For this review, take the finished solid that the model builds, in its own axes (mm). A direction names the side the tool comes from. Coordinates: 2 decimals unless noted, no trailing zeros. Loops run counter-clockwise (first coordinate to the right, second up) from the corner with the lowest first, then second, coordinate; pieces in that order, holes last. Notation, with made-up numbers: (-8, 84.5) - (-1, 84.5) arc R19 cw to (-1, 98.5) - close; hole circle Ø8 at (-4, 61.25). An arc over 180 degrees is marked (long way). Use one line per item in the form item = value. Start each with the question number.
1. Machinability: for faces 5 (the face through (6.762, -14, 1)), 6 (the face through (7.649, -13, 1)), 7 (the face through (5, 26, 1)), which of the approach directions +Z, -Z, +X, -X, +Y, -Y give a long, thin tool a straight path to every point of the face, cutting with its end or side? Answer none if there is none.
2. Add section B-B on y = 7. Give the boundary of the cut face in (x, z).
3. Draft analysis for pull direction X (two halves, no side actions). For faces 1 (the face through (5, -8, 1)), 2 (the face through (-42.81, -0.96, 1.48)), 3 (the face through (0, -46, 1)), 4 (the face through (-45.5, 0, 1)), state which applies: +X half, -X half, draft (parallel to the pull), parting line (faces both ways), or undercut.
4. For pin 1 Ø1.5 at (y, z) = (-14.5, 2) entering from -X; pin 2 Ø1.5 at (x, z) = (-25.5, 1.5) entering from -Y; pin 3 Ø6 at (x, y) = (-13, 6.5) entering from -Z; pin 4 Ø4 at (x, y) = (-40.5, 0) entering from +Z, all flat-tipped, find the tip position at first contact; note any pin that passes through.
5. Add section A-A on x = -40.5. Give the boundary of the cut face in (y, z), and give its area (3 significant figures).
6. Add section C-C on z = 0.6. Count the separate pieces of the cut face and the enclosed holes in it, and give its area (3 significant figures).
7. To check wall thickness, follow probe 1 along X at (y, z) = (42, 0.75); probe 2 along X at (y, z) = (7.5, 1.75). State the ranges of each line that lie inside material, in increasing order.
```python
from build123d import *

# Parameters (mm, degrees)
F0_R     = 2.5
F1_DEPTH = 3


with BuildPart() as f1:
    # F0 (on Top) → F1 (new body)
    with BuildSketch(Plane.XY):
        Polygon((5, 47), (0, 47), (-5, 47), (-5, 5), (-45.5, 5), (-45.5, 0), (-45.5, -5), (-5, -5), (-5, -46), (0, -46), (5, -46), (5, -10.4356960682), (4.7629147731, -10.1287784653), (5, -9.9454247125), (5, -5), (46.5, -5), (46.5, 0), (46.5, 5), (5, 5), align=None)
        with BuildLine():
            ThreePointArc((2.5, -41), (1.767766953, -42.767766953), (0, -43.5))
            ThreePointArc((0, -43.5), (-1.767766953, -39.232233047), (2.5, -41))
        make_face(mode=Mode.SUBTRACT)
        with BuildLine():
            ThreePointArc((-38, 0), (-40.5, -2.5), (-43, 0))
            ThreePointArc((-43, 0), (-40.5, 2.5), (-38, 0))
        make_face(mode=Mode.SUBTRACT)
        with BuildLine():
            ThreePointArc((2.5, 0), (-2.3096988313, -0.9567085809), (1.767766953, 1.767766953))
            ThreePointArc((1.767766953, 1.767766953), (2.3096988313, 0.9567085809), (2.5, 0))
        make_face(mode=Mode.SUBTRACT)
        Polygon((3.5076020164, -13.8316004514), (3.5076020164, -14.659125062), (2.3189120038, -14.659125062), (2.3189120038, -16.5000166744), (1.4475566406, -16.5000166744), (1.4475566406, -14.659125062), (-2.4481206573, -14.659125062), (-2.4481206573, -13.8649118235), (1.3546354449, -8.4456775625), (2.3189120038, -8.4456775625), (2.3189120038, -13.8316004514), align=None, mode=Mode.SUBTRACT)
        Polygon((9.3614297288, -0.567920358), (9.3614297288, -0.9107060472), (8.869038421, -0.9107060472), (8.869038421, -1.6732589575), (8.5080967101, -1.6732589575), (8.5080967101, -0.9107060472), (6.8943895038, -0.9107060472), (6.8943895038, -0.5817189344), (8.4696059442, 1.6630915853), (8.869038421, 1.6630915853), (8.869038421, -0.567920358), align=None, mode=Mode.SUBTRACT)
        with BuildLine():
            Line((11.0768106565, 1.6449355636), (11.0768106565, -1.6732589575))
            Line((11.0768106565, -1.6732589575), (10.7093327779, -1.6732589575))
            Line((10.7093327779, -1.6732589575), (10.7093327779, 0.6913813053))
            add(Edge.make_bspline(
                [(10.7093327779, 0.6913813053), (10.7093327779, 0.9869613382), (10.7274887995, 1.249860532)],
                knots=[0, 0, 0, 1, 1, 1], degree=2))
            add(Edge.make_bspline(
                [(10.7274887995, 1.249860532), (10.6802831432, 1.2019286348), (10.6210945125, 1.1500024128)],
                knots=[0, 0, 0, 1, 1, 1], degree=2))
            add(Edge.make_bspline(
                [(10.6210945125, 1.1500024128), (10.5619058819, 1.0980761908), (10.0811344279, 0.7073586044)],
                knots=[0, 0, 0, 1, 1, 1], degree=2))
            Line((10.0811344279, 0.7073586044), (9.8814181895, 0.965900353))
            Line((9.8814181895, 0.965900353), (10.7594433977, 1.6449355636))
            Line((10.7594433977, 1.6449355636), (11.0768106565, 1.6449355636))
        make_face(mode=Mode.SUBTRACT)
        with BuildLine():
            add(Edge.make_bspline(
                [(12.5325604743, -1.667812151), (12.4566683037, -1.5962774256), (12.4566683037, -1.4328732305)],
                knots=[0, 0, 0, 1, 1, 1], degree=2))
            add(Edge.make_bspline(
                [(12.4566683037, -1.4328732305), (12.4566683037, -1.2803626484), (12.5260243065, -1.2022917552)],
                knots=[0, 0, 0, 1, 1, 1], degree=2))
            add(Edge.make_bspline(
                [(12.5260243065, -1.2022917552), (12.5953803093, -1.124220862), (12.7246511836, -1.124220862)],
                knots=[0, 0, 0, 1, 1, 1], degree=2))
            add(Edge.make_bspline(
                [(12.7246511836, -1.124220862), (12.8561007806, -1.124220862), (12.9298142286, -1.2022917552)],
                knots=[0, 0, 0, 1, 1, 1], degree=2))
            add(Edge.make_bspline(
                [(12.9298142286, -1.2022917552), (13.0035276766, -1.2803626484), (13.0035276766, -1.4328732305)],
                knots=[0, 0, 0, 1, 1, 1], degree=2))
            add(Edge.make_bspline(
                [(13.0035276766, -1.4328732305), (13.0035276766, -1.5803001265), (12.9287248673, -1.6598235014)],
                knots=[0, 0, 0, 1, 1, 1], degree=2))
            add(Edge.make_bspline(
                [(12.9287248673, -1.6598235014), (12.853922058, -1.7393468763), (12.7246511836, -1.7393468763)],
                knots=[0, 0, 0, 1, 1, 1], degree=2))
            add(Edge.make_bspline(
                [(12.7246511836, -1.7393468763), (12.6084526449, -1.7393468763), (12.5325604743, -1.667812151)],
                knots=[0, 0, 0, 1, 1, 1], degree=2))
        make_face(mode=Mode.SUBTRACT)
        with BuildLine():
            add(Edge.make_bspline(
                [(14.092888977, 0.3013899598), (14.3536094482, 0.3536793022), (14.6128774377, 0.3536793022)],
                knots=[0, 0, 0, 1, 1, 1], degree=2))
            add(Edge.make_bspline(
                [(14.6128774377, 0.3536793022), (15.1372233437, 0.3536793022), (15.4378870626, 0.0936850718)],
                knots=[0, 0, 0, 1, 1, 1], degree=2))
            add(Edge.make_bspline(
                [(15.4378870626, 0.0936850718), (15.7385507815, -0.1663091585), (15.7385507815, -0.6180309778)],
                knots=[0, 0, 0, 1, 1, 1], degree=2))
            add(Edge.make_bspline(
                [(15.7385507815, -0.6180309778), (15.7385507815, -1.1329357524), (15.4106530301, -1.4259739423)],
                knots=[0, 0, 0, 1, 1, 1], degree=2))
            add(Edge.make_bspline(
                [(15.4106530301, -1.4259739423), (15.0827552786, -1.7190121321), (14.5061200303, -1.7190121321)],
                knots=[0, 0, 0, 1, 1, 1], degree=2))
            add(Edge.make_bspline(
                [(14.5061200303, -1.7190121321), (13.945462081, -1.7190121321), (13.650608289, -1.5396306379)],
                knots=[0, 0, 0, 1, 1, 1], degree=2))
            Line((13.650608289, -1.5396306379), (13.650608289, -1.1765102045))
            add(Edge.make_bspline(
                [(13.650608289, -1.1765102045), (13.808928798, -1.2781839258), (14.0449570798, -1.3362831952)],
                knots=[0, 0, 0, 1, 1, 1], degree=2))
            add(Edge.make_bspline(
                [(14.0449570798, -1.3362831952), (14.2809853615, -1.3943824645), (14.5104774755, -1.3943824645)],
                knots=[0, 0, 0, 1, 1, 1], degree=2))
            add(Edge.make_bspline(
                [(14.5104774755, -1.3943824645), (14.9099099523, -1.3943824645), (15.1310502963, -1.2059229596)],
                knots=[0, 0, 0, 1, 1, 1], degree=2))
            add(Edge.make_bspline(
                [(15.1310502963, -1.2059229596), (15.3521906403, -1.0174634546), (15.3521906403, -0.6608791889)],
                knots=[0, 0, 0, 1, 1, 1], degree=2))
            add(Edge.make_bspline(
                [(15.3521906403, -0.6608791889), (15.3521906403, 0.0334070799), (14.5017625851, 0.0334070799)],
                knots=[0, 0, 0, 1, 1, 1], degree=2))
            add(Edge.make_bspline(
                [(14.5017625851, 0.0334070799), (14.2860690476, 0.0334070799), (13.9251273367, -0.032680839)],
                knots=[0, 0, 0, 1, 1, 1], degree=2))
            Line((13.9251273367, -0.032680839), (13.7297685435, 0.0922325901))
            Line((13.7297685435, 0.0922325901), (13.8546819726, 1.6449355636))
            Line((13.8546819726, 1.6449355636), (15.5047012223, 1.6449355636))
            Line((15.5047012223, 1.6449355636), (15.5047012223, 1.2977924292))
            Line((15.5047012223, 1.2977924292), (14.1771329175, 1.2977924292))
            Line((14.1771329175, 1.2977924292), (14.092888977, 0.3013899598))
        make_face(mode=Mode.SUBTRACT)
        with Locations((41.5, 0)):
            Circle(F0_R, mode=Mode.SUBTRACT)
        with BuildLine():
            ThreePointArc((0, 44.5), (1.767766953, 43.767766953), (2.5, 42))
            ThreePointArc((2.5, 42), (-1.767766953, 40.232233047), (0, 44.5))
        make_face(mode=Mode.SUBTRACT)
        with BuildLine():
            Line((6.8825699725, -8.4895083152), (5, -9.9454247125))
            Line((5, -9.9454247125), (5, -10.4356960682))
            Line((5, -10.4356960682), (5.2450530525, -10.7529283834))
            add(Edge.make_bspline(
                [(6.5485796371, -9.6843346332), (6.4056913834, -9.8096905858), (5.2450530525, -10.7529283834)],
                knots=[0, 0, 0, 1, 1, 1], degree=2))
            add(Edge.make_bspline(
                [(6.8054278478, -9.4432654934), (6.6914678909, -9.5589786805), (6.5485796371, -9.6843346332)],
                knots=[0, 0, 0, 1, 1, 1], degree=2))
            add(Edge.make_bspline(
                [(6.7615970951, -10.7914994458), (6.7615970951, -10.0779347922), (6.8054278478, -9.4432654934)],
                knots=[0, 0, 0, 1, 1, 1], degree=2))
            Line((6.7615970951, -10.7914994458), (6.7615970951, -16.5000166744))
            Line((6.7615970951, -16.5000166744), (7.6487315293, -16.5000166744))
            Line((7.6487315293, -16.5000166744), (7.6487315293, -8.4895083152))
            Line((7.6487315293, -8.4895083152), (6.8825699725, -8.4895083152))
        make_face()
        Polygon((5, -10.4356960682), (5, -9.9454247125), (4.7629147731, -10.1287784653), align=None)
    extrude(amount=F1_DEPTH)


solid = f1.part
```
Conclusion:
q1.face_5 = +Z, -Z, -Y
q1.face_6 = +Z, -Z, +X, -Y
q1.face_7 = +Z, -Z, +X, +Y
q2.outline = (-5, 0) - (5, 0) - (5, 3) - (-5, 3) - close
q3.face_1 = undercut
q3.face_2 = undercut
q3.face_3 = draft
q3.face_4 = -X half
q4.pin_1 = -5
q4.pin_2 = -5
q4.pin_3 = 0
q4.pin_4 = through
q5.outline = (-5, 0) - (-2.5, 0) - (-2.5, 3) - (-5, 3) - close; (2.5, 0) - (5, 0) - (5, 3) - (2.5, 3) - close
q5.area = 15.0 mm^2
q6.separate_pieces = 1
q6.enclosed_holes = 10
q6.area = 1,630 mm^2
q7.probe_1 = -5 to -2.5, 2.5 to 5
q7.probe_2 = -5 to 5
